CAD build for the part. Positions are in the model's coordinates, mm. A direction names the side the tool comes from. Coordinates: 2 decimals unless noted, no trailing zeros. Loops run counter-clockwise (first coordinate to the right, second up) from the corner with the lowest first, then second, coordinate; pieces in that order, holes last. Notation, with made-up numbers: (-34.75, 4.25) -> (19.25, 4.25) arc R18 ccw to (19.25, 30.25) -> close; hole circle Ø7 at (-36, 88.25). An arc over 180 degrees is marked (long way). Return JSON: item names as keys, results as strings. Group by question number.
(1) Flat gauge pins, fed straight in: pin 1 Ø4.5 at (x, z) = (31.75, 0) entering from +Y; pin 2 Ø5.5 at (x, z) = (31.75, -19.05) entering from -Y; pin 3 Ø4.5 at (x, z) = (-31.75, 19.05) entering from -Y; pin 4 Ø10 at (x, z) = (-12.5, 4.5) entering from +Y. Where does each tip first touch, or does it go through?
(2) Saw through at A-A on z = 0. Write the cut outline in (x, y), then the cut area to 3 significant figures.
(3) Probe L1, parallel to X at y = 4.25, z = 13; L2, parallel to Z at x = 31.75, y = 3.7 (3 decimals); L3, parallel to Z at x = -31.75, y = 7. List the from-to ranges inside material, lowest first.
(4) Mould opens along X. For faces 4 (the face through (-36.492, 6.519, -23.833)), 5 (the face through (-20.028, 7.879, 15.352)), 6 (the face through (36.533, 6.519, 23.792)), 7 (the face through (0, 2.921, 0)) say: pulls with the +X half, pulls with the -X half, needs draft (parallel to the pull), parting line crosses it, or undercut.
(5) Saw through at B-B on x = 0. Write the cut outline in (y, z), then the cut area to 3 significant figures.
(6) Saw through at C-C on x = 31.75. Give the number of separate pieces and of enclosed holes in the cut face, then the cut area to 3 significant figures.
(7) Tool access for faces 1 (the face through (29.083, 8, 11)), 2 (the face through (-0.44, 6.44, -17.08)), 3 (the face through (-27.644, 2.762, -20.752)): list every direction of +Z, -Z, +X, -X, +Y, -Y with a clear straight run to the whole face (end or side of a thin tool).
```python
from build123d import *

# Parameters (mm, degrees)
SKETCH1_W                                      = 76.2
SKETCH1_H                                      = 50.8
BOSS_EXTRUDE1_DEPTH                            = 12.7
SKETCH2_W                                      = 51.308
SKETCH2_H                                      = 25.908
CUT_EXTRUDE1_DEPTH                             = 9.779
CUT_EXTRUDE2_DEPTH                             = 9.779
MIRROR2_COPY_1_DEPTH                           = 9.779
CBORE_FOR_10_SOCKET_HEAD_CAP_SCREW_D           = 4.9784
CBORE_FOR_10_SOCKET_HEAD_CAP_SCREW_CBORE_D     = 8.89
CBORE_FOR_10_SOCKET_HEAD_CAP_SCREW_CBORE_DEPTH = 5.08
CHAMFER1_SIZE                                  = 3.175
FILLET1_R                                      = 0.508
CHAMFER2_SIZE                                  = 0.508
F_10_32_TAPPED_HOLE1_D                         = 4.0386
CHAMFER3_SIZE                                  = 0.508


with BuildPart() as part:
    # Sketch1 → Boss-Extrude1 (new body)
    with BuildSketch(Plane(origin=(0, 0, 0), x_dir=(1, 0, 0), z_dir=(0, 1, 0))):
        Rectangle(SKETCH1_W, SKETCH1_H)
    extrude(amount=BOSS_EXTRUDE1_DEPTH)

    # Sketch2 → Cut-Extrude1 (cut)
    with BuildSketch(Plane(origin=(0, 12.7, 0), x_dir=(1, 0, 0), z_dir=(0, 1, 0))):
        Rectangle(SKETCH2_W, SKETCH2_H)
    extrude(amount=-CUT_EXTRUDE1_DEPTH, mode=Mode.SUBTRACT)

    # Sketch3 → Cut-Extrude2 (cut)
    with BuildSketch(Plane(origin=(0, 12.7, 0), x_dir=(1, 0, 0), z_dir=(0, 1, 0))):
        with BuildLine():
            Line((-22.479, 16.383), (-25.654, 16.383))
            ThreePointArc((-25.654, 16.383), (-28.078669153, 15.378669153), (-29.083, 12.954))
            Line((-29.083, 12.954), (-29.083, 9.779))
            ThreePointArc((-29.083, 9.779), (-26.96622149, 6.611017083), (-23.229330847, 7.354330847))
            Line((-23.229330847, 7.354330847), (-20.054330847, 10.529330847))
            ThreePointArc((-20.054330847, 10.529330847), (-19.311017083, 14.26622149), (-22.479, 16.383))
        make_face()
    cut_extrude2 = extrude(amount=-CUT_EXTRUDE2_DEPTH, mode=Mode.SUBTRACT)

    # Mirror1: Cut-Extrude2 across plane
    add(cut_extrude2.mirror(Plane.XY), mode=Mode.SUBTRACT)

    # Mirror2: Cut-Extrude2 across plane
    add(cut_extrude2.mirror(Plane(origin=(0, 0, 0), x_dir=(0, 0, 1), z_dir=(1, 0, 0))), mode=Mode.SUBTRACT)

    # Mirror2 copy 1 sketch → Mirror2 copy 1 (cut)
    with BuildSketch(Plane(origin=(0, 12.7, 0), x_dir=(-1, 0, 0), z_dir=(0, 1, 0))):
        with BuildLine():
            Line((-22.479, 16.383), (-25.654, 16.383))
            ThreePointArc((-25.654, 16.383), (-28.078669153, 15.378669153), (-29.083, 12.954))
            Line((-29.083, 12.954), (-29.083, 9.779))
            ThreePointArc((-29.083, 9.779), (-26.96622149, 6.611017083), (-23.229330847, 7.354330847))
            Line((-23.229330847, 7.354330847), (-20.054330847, 10.529330847))
            ThreePointArc((-20.054330847, 10.529330847), (-19.311017083, 14.26622149), (-22.479, 16.383))
        make_face()
    extrude(amount=-MIRROR2_COPY_1_DEPTH, mode=Mode.SUBTRACT)

    # CBORE for #10 Socket Head Cap Screw (through all)
    with Locations(Plane(origin=(-13.395092078, 0, 69.634435184), x_dir=(1, 0, 0), z_dir=(0, -1, 0))):
        with Locations((-18.354907922, -50.584435184), (45.145092078, -50.584435184), (45.145092078, -88.684435184), (-18.354907922, -88.684435184)):
            CounterBoreHole(CBORE_FOR_10_SOCKET_HEAD_CAP_SCREW_D / 2, CBORE_FOR_10_SOCKET_HEAD_CAP_SCREW_CBORE_D / 2, CBORE_FOR_10_SOCKET_HEAD_CAP_SCREW_CBORE_DEPTH)

    # Chamfer1
    chamfer1_edges = [part.edges().sort_by_distance(p)[0] for p in [
        (38.1, 6.35, 25.4),
        (-38.1, 6.35, 25.4),
        (-38.1, 6.35, -25.4),
        (38.1, 6.35, -25.4),
    ]]
    chamfer(chamfer1_edges, length=CHAMFER1_SIZE)

    # Fillet1
    fillet1_edges = [part.edges().sort_by_distance(p)[0] for p in [
        (38.1, 6.35, -22.225),
        (38.1, 6.35, 22.225),
        (-34.925, 6.35, 25.4),
        (34.925, 6.35, 25.4),
        (-34.925, 6.35, -25.4),
        (34.925, 6.35, -25.4),
        (-38.1, 6.35, -22.225),
        (-38.1, 6.35, 22.225),
    ]]
    fillet(fillet1_edges, radius=FILLET1_R)

    # Chamfer2
    chamfer2_edges = [part.edges().sort_by_distance(p)[0] for p in [
        (-38.1, 0, 0),
        (38.1, 0, 0),
        (36.5125, 0, 23.8125),
        (0, 0, 25.4),
        (-36.5125, 0, 23.8125),
        (-36.5125, 0, -23.8125),
        (0, 0, -25.4),
        (36.5125, 0, -23.8125),
        (-34.908982694, 0, 25.361330803),
        (-38.061330803, 0, 22.208982694),
        (34.908982694, 0, 25.361330803),
        (38.061330803, 0, 22.208982694),
        (38.061330803, 0, -22.208982694),
        (34.908982694, 0, -25.361330803),
        (-34.908982694, 0, -25.361330803),
        (-38.061330803, 0, -22.208982694),
    ]]
    chamfer(chamfer2_edges, length=CHAMFER2_SIZE)

    # #10-32 Tapped Hole1 (through all)
    with Locations(Plane(origin=(0, 0, 0), x_dir=(-1, 0, 0), z_dir=(0, -1, 0))):
        with Locations((-31.75, 0), (31.75, 0), (0, 19.05), (0, -19.05)):
            Hole(F_10_32_TAPPED_HOLE1_D / 2)

    # Chamfer3
    chamfer3_edges = [part.edges().sort_by_distance(p)[0] for p in [
        (-36.195, 0, -19.05),
        (27.305, 0, -19.05),
        (27.305, 0, 19.05),
        (-36.195, 0, 19.05),
    ]]
    chamfer(chamfer3_edges, length=CHAMFER3_SIZE)


solid = part.part
```
Geometry results:
{
 "1": {"pin 1": "y = 12.7", "pin 2": "y = 5.08", "pin 3": "through", "pin 4": "y = 2.92"},
 "2": {"outline": "(-38.1, 0.51) -> (-37.59, 0) -> (-33.77, 0) -> (-33.77, 12.7) -> (-38.1, 12.7) -> close; (-29.73, 0) -> (29.73, 0) -> (29.73, 12.7) -> (25.65, 12.7) -> (25.65, 2.92) -> (-25.65, 2.92) -> (-25.65, 12.7) -> (-29.73, 12.7) -> close; (33.77, 0) -> (37.59, 0) -> (38.1, 0.51) -> (38.1, 12.7) -> (33.77, 12.7) -> close", "area": "363 mm²"},
 "3": {"L1": "-38.1 to -29.08, -19.05 to 19.05, 29.08 to 38.1", "L2": "-25.4 to -23.495, -14.605 to -2.019, 2.019 to 14.605, 23.495 to 25.4", "L3": "-25.4 to -21.54, -16.56 to -2.02, 2.02 to 16.56, 21.54 to 25.4"},
 "4": {"face 4": "pulls with the -X half", "face 5": "undercut", "face 6": "pulls with the +X half", "face 7": "undercut"},
 "5": {"outline": "(0, -24.89) -> (0.51, -25.4) -> (12.7, -25.4) -> (12.7, -21.07) -> (0, -21.07) -> close; (0, -17.03) -> (12.7, -17.03) -> (12.7, -12.95) -> (2.92, -12.95) -> (2.92, 12.95) -> (12.7, 12.95) -> (12.7, 17.03) -> (0, 17.03) -> close; (0, 21.07) -> (12.7, 21.07) -> (12.7, 25.4) -> (0.51, 25.4) -> (0, 24.89) -> close", "area": "289 mm²"},
 "6": {"separate pieces": "4", "enclosed holes": "0", "area": "427 mm²"},
 "7": {"face 1": "+Y", "face 2": "+Y, -Y", "face 3": "-Y"}
}
